Check sheet for the drawn part. Datum: minimum x, y, z corner. Units: mm. A direction names the side the tool comes from. Round coordinates to 2 decimals unless told otherwise and drop trailing zeros. Order: outer loops, then holes, each group sorted by start corner. A loop starts at its lowest first (then second) coordinate and runs counter-clockwise, first axis right, second up.
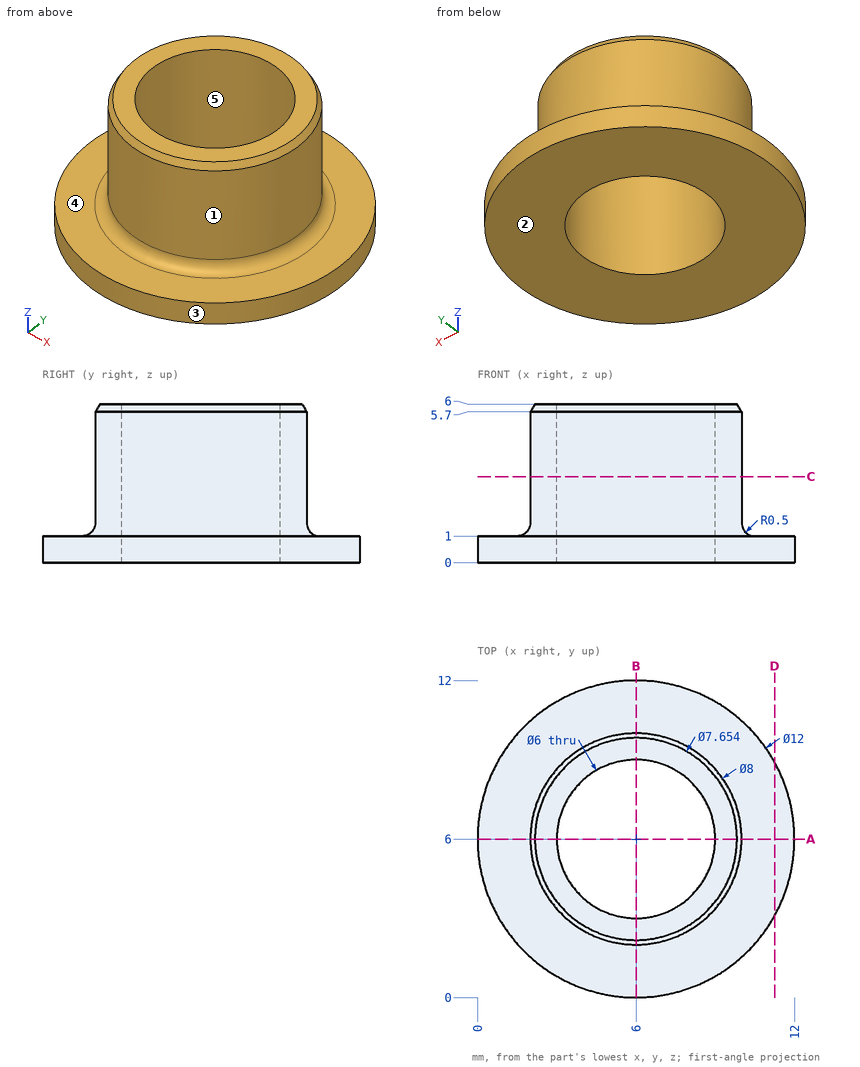
(1) Sectioned sample at C-C, the plane z = 3.25. Record the cut outline in (x, y), and give its area (3 significant figures).
Returned:
outline: circle Ø8 at (6, 6); hole circle Ø6 at (6, 6)
area: 22.0 mm2
(2) Sectioned sample at A-A, the plane y = 6. Record the cut outline in (x, z).
Returned:
outline: (0, 0) - (3, 0) - (3, 6) - (2.17, 6) - (2, 5.7) - (2, 1.5) arc R0.5 cw to (1.5, 1) - (0, 1) - close; (9, 0) - (12, 0) - (12, 1) - (10.5, 1) arc R0.5 cw to (10, 1.5) - (10, 5.7) - (9.83, 6) - (9, 6) - close
(3) Material ranges on line 1 (Y direction, x = 6, z = 2.1); line 2 (Z direction, x = 5, y = 11); line 3 (X direction, y = 5, z = 3.7), recorded low to high.
Returned:
line 1: y = 2 to 3, 9 to 10
line 2: z = 0 to 1
line 3: x = 2.13 to 3.17, 8.83 to 9.87
(4) Sectioned sample at D-D, the plane x = 11.25. Record the cut outline in (y, z) (1 decimal).
Returned:
outline: (3.1, 0) - (8.9, 0) - (8.9, 1) - (3.1, 1) - close
(5) Set-up check for the marked faces 1 and 2: record each of +Z, -Z, +X, -X, +Y, -Y from which the full face is reachable in a straight line by a thin tool's end or side.
Returned:
face 1: +Z
face 2: -Z, +X, -X, +Y, -Y
(6) Depth check by flat-ended pin: P1, Ø1, axis at x = 1, z = 4, coming from the -Y side. Enter the tip coordinate at first touch or a pass-through.
Returned:
P1: passes through
(7) Draft check along Y on the marked faces 3, 4 and 5. Enter one of: released by +Y, released by -Y, zero draft, split by the parting line, or undercut.
Returned:
face 3: split by the parting line
face 4: zero draft
face 5: undercut
